Design review of the part built by this model. Coordinates are the model's own, in mm. A direction names the side the tool comes from. Coordinates: 2 decimals unless noted, no trailing zeros. Loops run counter-clockwise (first coordinate to the right, second up) from the corner with the lowest first, then second, coordinate; pieces in that order, holes last. Notation, with made-up numbers: (-18.75, -1) - (32.25, -1) arc R35 cw to (32.25, 38) - close; hole circle Ø2 at (20.5, 87.25). An arc over 180 degrees is marked (long way). Answer in a Markdown table with one row per item. Add a question column.
(1) The part is to be moulded in two halves that separate along X. For faces 1 (the face through (0.53, 12.59, 0.59)), 2 (the face through (-4, -9, 0)), 3 (the face through (-1, -10, 1)), 4 (the face through (0, 10, 1)), say which applies: released by +X, released by -X, zero draft, split by the parting line, or undercut.
(2) For faces 5 (the face through (-4, -9, 1.2)), 6 (the face through (1, -10, 1)), 7 (the face through (3, -8.2, 1)), list the 3-axis set-ups (+Z, -Z, +X, -X, +Y, -Y) from which the entire face can be reached by the end or side of a thin tool; tool diameter is ignored.
(3) We need section B-B, the plane x = 2.5. Write out the cut boundary in (y, z), plus the area to 3 significant figures.
(4) We need section D-D, the plane z = 1. Give the number of separate pieces and of enclosed holes in the cut face, plus the area to 3 significant figures.
(5) We need section C-C, the plane x = 6.75. Write out the cut boundary in (y, z), plus the area to 3 significant figures.
(6) To check wall thickness, follow L1, parallel to X at y = 0, z = 0.9; L2, parallel to X at y = -10, z = 0.1; L3, parallel to Y at x = -2.5, z = 0.95. State the ranges of each line that lie inside material, in increasing order. Write a range as [from, to].
(7) Clearance check with flat-ended pins moving along their axes: pin 1 (3 mm diameter, centred on x = 4, y = 6.5, fed in from -Z); pin 2 (0.6 mm diameter, centred on x = 3, z = 0.5, fed in from +Y). State where each tip first meets the part, or that it passes through.
(8) We need section A-A, the plane y = 0. Write out the cut boundary in (x, z).
from build123d import *

# Parameters (mm, degrees)
SZKIC1_R                    = 1
DODANIE_WYCI_GNI_CIE1_DEPTH = 1.2
ZAOKR_GLENIE2_R             = 0.5
ZAOKR_GLENIE3_R             = 0.5
ZAOKR_GLENIE4_R             = 0.5
ZAOKR_GLENIE5_R             = 0.5
ZAOKR_GLENIE6_R             = 0.5
ZAOKR_GLENIE7_R             = 0.5
ZAOKR_GLENIE8_R             = 0.5
ZAOKR_GLENIE9_R             = 0.5


with BuildPart() as part:
    # Szkic1 → Dodanie-wyciągnięcie1 (new body)
    with BuildSketch(Plane.XY):
        with BuildLine():
            Line((-1, -12.560254774), (-1, -8.2))
            Line((-1, -8.2), (-4, -8.2))
            Line((-4, -8.2), (-4, -9.16515139))
            ThreePointArc((-4, -9.16515139), (0, 10), (4, -9.16515139))
            Line((4, -9.16515139), (4, -8.2))
            Line((4, -8.2), (1, -8.2))
            Line((1, -8.2), (1, -12.560254774))
            ThreePointArc((1, -12.560254774), (0, 12.6), (-1, -12.560254774))
        make_face()
        with Locations((2.5, -9.7)):
            Circle(SZKIC1_R, mode=Mode.SUBTRACT)
        with Locations((-2.5, -9.7)):
            Circle(SZKIC1_R, mode=Mode.SUBTRACT)
    extrude(amount=DODANIE_WYCI_GNI_CIE1_DEPTH)

    # Zaokrąglenie2
    zaokr_glenie2_edges = [part.edges().sort_by_distance(p)[0] for p in [
        (1, -12.560254774, 0.6),
    ]]
    fillet(zaokr_glenie2_edges, radius=ZAOKR_GLENIE2_R)

    # Zaokrąglenie3
    zaokr_glenie3_edges = [part.edges().sort_by_distance(p)[0] for p in [
        (-1, -12.560254774, 0.6),
    ]]
    fillet(zaokr_glenie3_edges, radius=ZAOKR_GLENIE3_R)

    # Zaokrąglenie4
    zaokr_glenie4_edges = [part.edges().sort_by_distance(p)[0] for p in [
        (1, -8.2, 0.6),
    ]]
    fillet(zaokr_glenie4_edges, radius=ZAOKR_GLENIE4_R)

    # Zaokrąglenie5
    zaokr_glenie5_edges = [part.edges().sort_by_distance(p)[0] for p in [
        (4, -8.2, 0.6),
    ]]
    fillet(zaokr_glenie5_edges, radius=ZAOKR_GLENIE5_R)

    # Zaokrąglenie6
    zaokr_glenie6_edges = [part.edges().sort_by_distance(p)[0] for p in [
        (4, -9.16515139, 0.6),
    ]]
    fillet(zaokr_glenie6_edges, radius=ZAOKR_GLENIE6_R)

    # Zaokrąglenie7
    zaokr_glenie7_edges = [part.edges().sort_by_distance(p)[0] for p in [
        (-4, -8.2, 0.6),
    ]]
    fillet(zaokr_glenie7_edges, radius=ZAOKR_GLENIE7_R)

    # Zaokrąglenie8
    zaokr_glenie8_edges = [part.edges().sort_by_distance(p)[0] for p in [
        (-1, -8.2, 0.6),
    ]]
    fillet(zaokr_glenie8_edges, radius=ZAOKR_GLENIE8_R)

    # Zaokrąglenie9
    zaokr_glenie9_edges = [part.edges().sort_by_distance(p)[0] for p in [
        (-4, -9.16515139, 0.6),
    ]]
    fillet(zaokr_glenie9_edges, radius=ZAOKR_GLENIE9_R)


solid = part.part
Responses:
| question | item | result |
|---|---|---|
| 1 | face 1 | split by the parting line |
| 1 | face 2 | zero draft |
| 1 | face 3 | undercut |
| 1 | face 4 | undercut |
| 2 | face 5 | +Z, +X, -X, +Y, -Y |
| 2 | face 6 | +Z, -Z, -Y |
| 2 | face 7 | +Z, -Z |
| 3 | outline | (-12.35, 0) - (-10.7, 0) - (-10.7, 1.2) - (-12.35, 1.2) - close; (-8.7, 0) - (-8.2, 0) - (-8.2, 1.2) - (-8.7, 1.2) - close; (9.68, 0) - (12.35, 0) - (12.35, 1.2) - (9.68, 1.2) - close |
| 3 | area | 5.78 mm2 |
| 4 | separate pieces | 1 |
| 4 | enclosed holes | 2 |
| 4 | area | 182 mm2 |
| 5 | outline | (-10.64, 0) - (-7.38, 0) - (-7.38, 1.2) - (-10.64, 1.2) - close; (7.38, 0) - (10.64, 0) - (10.64, 1.2) - (7.38, 1.2) - close |
| 5 | area | 7.83 mm2 |
| 6 | L1 | x = [-12.6, -10], [10, 12.6] |
| 6 | L2 | x = [-7.67, -3.45], [-1.55, -1], [1, 1.55], [3.45, 7.67] |
| 6 | L3 | y = [-12.35, -10.7], [-8.7, -8.2], [9.68, 12.35] |
| 7 | pin 1 | passes through |
| 7 | pin 2 | stops at y = 12.31 |
| 8 | outline | (-12.6, 0) - (-10, 0) - (-10, 1.2) - (-12.6, 1.2) - close; (10, 0) - (12.6, 0) - (12.6, 1.2) - (10, 1.2) - close |
